```python
from build123d import *

# Parameters (mm, degrees)
F0_W     = 73.482446
F0_H     = 70.119202
F1_DEPTH = 5
F2_T     = -2.5
F4_D     = 5


with BuildPart() as f1:
    # F0 (on Top) → F1 (new body)
    with BuildSketch(Plane.XY):
        with Locations((36.741223, -35.059601)):
            Rectangle(F0_W, F0_H)
    extrude(amount=F1_DEPTH)

    # F2
    f2_openings = [f1.faces().sort_by_distance(p)[0] for p in [
        (36.741223, -35.059601, 5),
    ]]
    offset(amount=F2_T, openings=f2_openings)

    # F4 (through all)
    with Locations(Plane.XY.offset(2.5)):
        with Locations((10.154494, -6.421357)):
            Hole(F4_D / 2)


solid = f1.part
```
The listing builds one solid part. Answer for the finished solid, in the listing's coordinates (mm). A direction names the side the tool comes from. Coordinates: 2 decimals unless noted, no trailing zeros. Write each loop counter-clockwise with the first axis right and the second up, starting at its lowest first coordinate (ties: lowest second). Pieces come first, ordered by that corner, then holes.
Q1. Given P1, Ø4, axis at x = 14, y = -13, coming from the +Z side, flat-ended and moving along its own axis, determine where the tip first touches the part or whether it passes through.
Returned:
P1: stops at z = 2.5
Q2. Which of the six approach directions +Z, -Z, +X, -X, +Y, -Y give full straight-line access (tool end or side, diameter ignored) to faces 1 (the flat face through (36, -67.619, 4)), 2 (the flat face through (34, -69, 5))?
Returned:
face 1: +Z
face 2: +Z, +X, -X, +Y, -Y
Q3. Section D-D, the plane x = 9 is taken. Write down the section's boundary in (y, z), then the cut area to 3 significant figures.
Returned:
outline: (-70.12, 0) - (-8.64, 0) - (-8.64, 2.5) - (-67.62, 2.5) - (-67.62, 5) - (-70.12, 5) - close; (-4.2, 0) - (0, 0) - (0, 5) - (-2.5, 5) - (-2.5, 2.5) - (-4.2, 2.5) - close
area: 177 mm2
Q4. Section C-C, the plane y = -23.5 is taken. Write down the section's boundary in (x, z), then the cut area to 3 significant figures.
Returned:
outline: (0, 0) - (73.48, 0) - (73.48, 5) - (70.98, 5) - (70.98, 2.5) - (2.5, 2.5) - (2.5, 5) - (0, 5) - close
area: 196 mm2
Q5. Section A-A, the plane z = 3.85 is taken. Write down the section's boundary in (x, y), then the cut area to 3 significant figures.
Returned:
outline: (0, -70.12) - (73.48, -70.12) - (73.48, 0) - (0, 0) - close; hole (2.5, -67.62) - (70.98, -67.62) - (70.98, -2.5) - (2.5, -2.5) - close
area: 693 mm2
Q6. Section B-B, the plane x = 68.5 is taken. Write down the section's boundary in (y, z), then the cut area to 3 significant figures.
Returned:
outline: (-70.12, 0) - (0, 0) - (0, 5) - (-2.5, 5) - (-2.5, 2.5) - (-67.62, 2.5) - (-67.62, 5) - (-70.12, 5) - close
area: 188 mm2
Q7. Find the intervals of material crossed by line 1 along X through (y, z) = (-24, 3.35); line 2 along Y through (x, z) = (43.5, 4.5); line 3 along Z through (x, y) = (45, -64), in increasing order.
Returned:
line 1: x = 0 to 2.5, 70.98 to 73.48
line 2: y = -70.12 to -67.62, -2.5 to 0
line 3: z = 0 to 2.5
Q8. The mould has two halves that part along Y. Classify faces 3 (the flat face through (36, 0, 2)), 4 (the flat face through (73.482, -36, 2)), 5 (the flat face through (2.5, -36, 4)): released by +Y, released by -Y, zero draft, split by the parting line, or undercut.
Returned:
face 3: released by +Y
face 4: zero draft
face 5: undercut
